Part model, mm, in its own coordinate system. A direction names the side the tool comes from. Round coordinates to 2 decimals unless told otherwise and drop trailing zeros. Write each loop counter-clockwise with the first axis right and the second up, starting at its lowest first coordinate (ties: lowest second). Pieces come first, ordered by that corner, then holes.
```python
from build123d import *

# Parameters (mm, degrees)
SKETCH_3_RX     = 15
SKETCH_3_RY     = 10
SKETCH_3_RX_2   = 25
EXTRUDE_1_DEPTH = 10
SKETCH_3_3_RX   = 15
SKETCH_3_3_RY   = 10
SKETCH_3_3_RX_2 = 25
EXTRUDE_2_DEPTH = 60


with BuildPart() as part:
    # 草图3 → 凸台-拉伸1 (new body)
    with BuildSketch(Plane.XY):
        with BuildLine():
            Line((0, 0), (212, -16.559778275))
            Line((212, -16.559778275), (212, -84.849778275))
            ThreePointArc((212, -84.849778275), (205.303937337, -99.783138625), (189.699474868, -104.717027308))
            Line((189.699474868, -104.717027308), (138.935384383, -157.579407289))
            Line((138.935384383, -157.579407289), (138.935384383, -187.579407289))
            ThreePointArc((138.935384383, -187.579407289), (136.006452195, -194.650475101), (128.935384383, -197.579407289))
            Line((128.935384383, -197.579407289), (-9.047403236, -197.579407289))
            ThreePointArc((-9.047403236, -197.579407289), (-19.348164734, -194.722753304), (-26.706355093, -186.968838545))
            Line((-26.706355093, -186.968838545), (-68.22172539, -108.889782909))
            ThreePointArc((-68.22172539, -108.889782909), (-69.376331833, -103.631064432), (-67.636828751, -98.535834793))
            Line((-67.636828751, -98.535834793), (0, 0))
        make_face()
        with Locations(Location((-0.530483272, -110.497923763), (0, 0, -135))):
            Ellipse(SKETCH_3_RX, SKETCH_3_RY, mode=Mode.SUBTRACT)
        with Locations(Location((102, -68.15020742), (0, 0, 90))):
            Ellipse(SKETCH_3_RX_2, SKETCH_3_RY, mode=Mode.SUBTRACT)
        with BuildLine():
            Line((17, -12.920611137), (37, -12.920611137))
            ThreePointArc((37, -12.920611137), (47, -22.920611137), (37, -32.920611137))
            Line((37, -32.920611137), (17, -32.920611137))
            ThreePointArc((17, -32.920611137), (7, -22.920611137), (17, -12.920611137))
        make_face(mode=Mode.SUBTRACT)
        with BuildLine():
            Line((151.527534094, -43.292720139), (172.74073753, -64.505923575))
            ThreePointArc((172.74073753, -64.505923575), (172.74073753, -78.708178021), (158.538483084, -78.708178021))
            Line((158.538483084, -78.708178021), (137.325279648, -57.494974585))
            ThreePointArc((137.325279648, -57.494974585), (137.325279648, -43.292720139), (151.527534094, -43.292720139))
        make_face(mode=Mode.SUBTRACT)
        with BuildLine():
            ThreePointArc((31.188356134, -144.606315506), (50.439261207, -171.820683387), (83.625615961, -174.96472909))
            ThreePointArc((83.625615961, -174.96472909), (90.385321801, -160.953791328), (76.374384039, -154.194085489))
            ThreePointArc((76.374384039, -154.194085489), (61.462059159, -152.781305107), (52.811643866, -140.552499073))
            ThreePointArc((52.811643866, -140.552499073), (39.973091784, -131.767763424), (31.188356134, -144.606315506))
        make_face(mode=Mode.SUBTRACT)
    extrude(amount=EXTRUDE_1_DEPTH)

    # 草图3<3> → 凸台-拉伸2 (add)
    with BuildSketch(Plane.XY):
        with BuildLine():
            Line((0, 0), (212, -16.559778275))
            Line((212, -16.559778275), (212, -84.849778275))
            ThreePointArc((212, -84.849778275), (205.303937337, -99.783138625), (189.699474868, -104.717027308))
            Line((189.699474868, -104.717027308), (138.935384383, -157.579407289))
            Line((138.935384383, -157.579407289), (138.935384383, -187.579407289))
            ThreePointArc((138.935384383, -187.579407289), (136.006452195, -194.650475101), (128.935384383, -197.579407289))
            Line((128.935384383, -197.579407289), (-9.047403236, -197.579407289))
            ThreePointArc((-9.047403236, -197.579407289), (-19.348164734, -194.722753304), (-26.706355093, -186.968838545))
            Line((-26.706355093, -186.968838545), (-68.22172539, -108.889782909))
            ThreePointArc((-68.22172539, -108.889782909), (-69.376331833, -103.631064432), (-67.636828751, -98.535834793))
            Line((-67.636828751, -98.535834793), (0, 0))
        make_face()
        with Locations(Location((-0.530483272, -110.497923763), (0, 0, -135))):
            Ellipse(SKETCH_3_3_RX, SKETCH_3_3_RY, mode=Mode.SUBTRACT)
        with Locations(Location((102, -68.15020742), (0, 0, 90))):
            Ellipse(SKETCH_3_3_RX_2, SKETCH_3_3_RY, mode=Mode.SUBTRACT)
        with BuildLine():
            Line((17, -12.920611137), (37, -12.920611137))
            ThreePointArc((37, -12.920611137), (47, -22.920611137), (37, -32.920611137))
            Line((37, -32.920611137), (17, -32.920611137))
            ThreePointArc((17, -32.920611137), (7, -22.920611137), (17, -12.920611137))
        make_face(mode=Mode.SUBTRACT)
        with BuildLine():
            Line((151.527534094, -43.292720139), (172.74073753, -64.505923575))
            ThreePointArc((172.74073753, -64.505923575), (172.74073753, -78.708178021), (158.538483084, -78.708178021))
            Line((158.538483084, -78.708178021), (137.325279648, -57.494974585))
            ThreePointArc((137.325279648, -57.494974585), (137.325279648, -43.292720139), (151.527534094, -43.292720139))
        make_face(mode=Mode.SUBTRACT)
        with BuildLine():
            ThreePointArc((31.188356134, -144.606315506), (50.439261207, -171.820683387), (83.625615961, -174.96472909))
            ThreePointArc((83.625615961, -174.96472909), (90.385321801, -160.953791328), (76.374384039, -154.194085489))
            ThreePointArc((76.374384039, -154.194085489), (61.462059159, -152.781305107), (52.811643866, -140.552499073))
            ThreePointArc((52.811643866, -140.552499073), (39.973091784, -131.767763424), (31.188356134, -144.606315506))
        make_face(mode=Mode.SUBTRACT)
    extrude(amount=EXTRUDE_2_DEPTH)


solid = part.part
```
Q1. Cut at A-A on x = 21. Write the cut outline in (y, z), plus the area to 3 significant figures.
Values follow:
outline: (-197.58, 0) - (-32.92, 0) - (-32.92, 60) - (-197.58, 60) - close; (-12.92, 0) - (-1.64, 0) - (-1.64, 60) - (-12.92, 60) - close
area: 10,600 mm2
Q2. Cut at D-D on x = 118.5. Write the cut outline in (y, z), plus the area to 3 significant figures.
Values follow:
outline: (-197.58, 0) - (-9.26, 0) - (-9.26, 60) - (-197.58, 60) - close
area: 11,300 mm2
Q3. Drop flat-ended pins along their axis: pin 1 (10 mm diameter, centred on x = 22.5, z = 31, fed in from +Y); pin 2 (3 mm diameter, centred on y = -118.5, z = 42.5, fed in from +X); pin 3 (6 mm diameter, centred on x = 54, z = 25.5, fed in from +Y); pin 4 (4 mm diameter, centred on x = 97.5, y = -123, fed in from -Z). Give the stop position or say it passes through.
Values follow:
pin 1: stops at y = -1.37
pin 2: stops at x = 177.9
pin 3: stops at y = -3.98
pin 4: stops at z = 0
Q4. Mould opens along Y. For faces 4 (the cylindrical face through (50.024, -171.577, 29.58)), 5 (the flat face through (27, -32.921, 30)), 6 (the flat face through (104.516, -8.164, 29.58)), 7 (the cylindrical face through (-19.22, -194.8, 29.58)) say: +Y half, -Y half, draft (parallel to the pull), parting line (faces both ways), or undercut.
Values follow:
face 4: undercut
face 5: undercut
face 6: +Y half
face 7: -Y half
Q5. Cut at B-B on x = 60. Write the cut outline in (y, z).
Values follow:
outline: (-197.58, 0) - (-175.8, 0) - (-175.8, 60) - (-197.58, 60) - close; (-151.84, 0) - (-4.69, 0) - (-4.69, 60) - (-151.84, 60) - close
Q6. Wall check: L1, parallel to Y at x = 9, z = 10; L2, parallel to X at y = -65, z = 40.5; L3, parallel to X at y = -48, z = 6. Give the ranges that are in metal, low to high.
Values follow:
L1: y = -197.58 to -114.65, -99.02 to -28.92, -16.92 to -0.7
L2: x = -44.62 to 92.08, 111.92 to 144.83, 173.2 to 212
L3: x = -32.95 to 96.08, 107.92 to 134.67, 156.23 to 212
Q7. Cut at C-C on z = 27. State how many separate pieces and enclosed holes the cut face has, plus the area to 3 significant figures.
Values follow:
separate pieces: 1
enclosed holes: 5
area: 38,200 mm2
Q8. Which spindle directions (+Z, -Z, +X, -X, +Y, -Y) get a long thin tool onto all of the face, cutting with end or side? Do faces 1 (the cylindrical face through (61.65, -152.89, 29.58)), 2 (the cylindrical face through (-69.38, -103.71, 29.58)), 3 (the flat face through (138.935, -172, 30)). Say none if no direction does.
Values follow:
face 1: +Z, -Z
face 2: +Z, -Z, -X
face 3: +Z, -Z, +X, -Y
